Verification items for the finished model (mm, model axes). Face numbers are marked on the shaded views. Round coordinates to 2 decimals unless told otherwise and drop trailing zeros. Order: outer loops, then holes, each group sorted by start corner. A loop starts at its lowest first (then second) coordinate and runs counter-clockwise, first axis right, second up. Notation, with made-up numbers: (-16.5, 43.25) -> (-5.5, 43.25) arc R33 ccw to (-5.5, 79.25) -> close; hole circle Ø9 at (20, 20). An arc over 180 degrees is marked (long way). Put each result on its own line as item: value.
from build123d import *

# Parameters (mm, degrees)
F0_R     = 2.5
F1_DEPTH = 12.7
F2_DEPTH = 4


# Not quite as in the source:
# - a length typed as a fraction of an inch, garbled in the dataset ("3 / 203.2 mm" for 3/8 in), is restored
# - a feature names something its author has since deleted; it is built from what else it names


with BuildPart() as f1:
    # F0 (on Top) → F1 (new body)
    with BuildSketch(Plane.XY):
        Polygon((0, 60), (0, 0), (10, 0), (10, 50), (10, 56.35), (16.35, 56.35), (16.35, 50), (54.65, 50), (54.65, 56.35), (61, 56.35), (61, 50), (61, 0), (71, 0), (71, 60), align=None)
        Polygon((10, 50), (10, 0), (61, 0), (61, 50), (61, 56.35), (54.65, 56.35), (54.65, 50), (16.35, 50), (16.35, 56.35), (10, 56.35), align=None)
        with Locations((19.5, 43)):
            Circle(F0_R, mode=Mode.SUBTRACT)
        with Locations((51.5, 43)):
            Circle(F0_R, mode=Mode.SUBTRACT)
    extrude(amount=-F1_DEPTH)

    # F0 (on Top) → F2 (cut)
    with BuildSketch(Plane.XY):
        Polygon((10, 50), (10, 0), (61, 0), (61, 50), (61, 56.35), (54.65, 56.35), (54.65, 50), (16.35, 50), (16.35, 56.35), (10, 56.35), align=None)
        with Locations((19.5, 43)):
            Circle(F0_R, mode=Mode.SUBTRACT)
        with Locations((51.5, 43)):
            Circle(F0_R, mode=Mode.SUBTRACT)
    extrude(amount=-F2_DEPTH, mode=Mode.SUBTRACT)


solid = f1.part
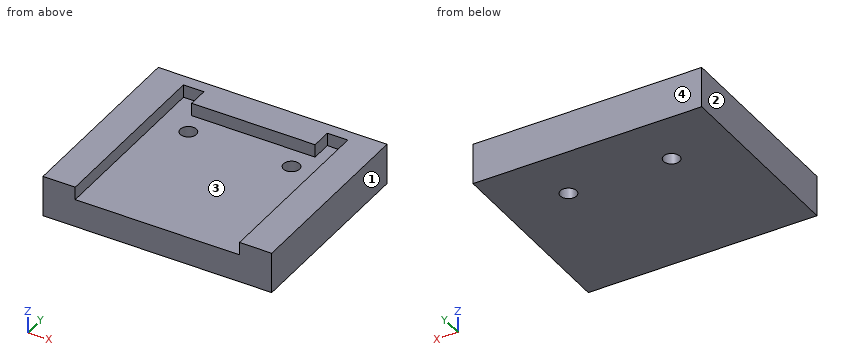
Item 1: Release check for a two-part mould opening along X. For the marked faces 1, 2, 3 and 4 record: +X half, -X half, draft (parallel to the pull), parting line (faces both ways), or undercut.
Check sheet entries:
face 1: +X half
face 2: -X half
face 3: undercut
face 4: draft
Item 2: Section check C-C on y = 10.5. Record the boundary of the cut face in (x, z), then the cut area to 3 significant figures.
Check sheet entries:
outline: (0, -12.7) -> (71, -12.7) -> (71, 0) -> (61, 0) -> (61, -4) -> (10, -4) -> (10, 0) -> (0, 0) -> close
area: 698 mm^2
Item 3: Material ranges on L1, parallel to X at y = 16, z = -0.75; L2, parallel to Y at x = 51.5, z = -6; L3, parallel to Z at x = 45.5, y = 12, recorded low to high. Write a range as [from, to].
Check sheet entries:
L1: x = [0, 10], [61, 71]
L2: y = [0, 40.5], [45.5, 60]
L3: z = [-12.7, -4]
Item 4: Section check D-D on y = 54. Record the boundary of the cut face in (x, z), then the cut area to 3 significant figures.
Check sheet entries:
outline: (0, -12.7) -> (71, -12.7) -> (71, 0) -> (61, 0) -> (61, -4) -> (54.65, -4) -> (54.65, 0) -> (16.35, 0) -> (16.35, -4) -> (10, -4) -> (10, 0) -> (0, 0) -> close
area: 851 mm^2
Item 5: Section check A-A on x = 19.5. Record the boundary of the cut face in (y, z).
Check sheet entries:
outline: (0, -12.7) -> (40.5, -12.7) -> (40.5, -4) -> (0, -4) -> close; (45.5, -12.7) -> (60, -12.7) -> (60, 0) -> (50, 0) -> (50, -4) -> (45.5, -4) -> close
Item 6: Gauge pin test, flat ends, axial feed: pin 1 Ø2 at (x, z) = (57.5, -1) entering from -Y; pin 2 Ø1.5 at (x, y) = (14, 11) entering from +Z; pin 3 Ø1.2 at (x, z) = (40.5, -2) entering from -Y. Record the tip position at first contact, or that the pin passes through.
Check sheet entries:
pin 1: stops at y = 56.35
pin 2: stops at z = -4
pin 3: stops at y = 50
Item 7: Section check B-B on y = 43. Record the boundary of the cut face in (x, z).
Check sheet entries:
outline: (0, -12.7) -> (17, -12.7) -> (17, -4) -> (10, -4) -> (10, 0) -> (0, 0) -> close; (22, -12.7) -> (49, -12.7) -> (49, -4) -> (22, -4) -> close; (54, -12.7) -> (71, -12.7) -> (71, 0) -> (61, 0) -> (61, -4) -> (54, -4) -> close
